from build123d import *

# Parameters (mm, degrees)
SKETCH1_R           = 5.2575
BOSS_EXTRUDE2_DEPTH = 18.3
SKETCH3_R           = 1.75
CUT_EXTRUDE2_DEPTH  = 19.8
SKETCH4_R           = 5.2575
SKETCH4_R_2         = 3.5
CUT_EXTRUDE3_DEPTH  = 16.5
FILLET1_R           = 0.5
FILLET2_R           = 0.25
FILLET3_R           = 0.5


with BuildPart() as part:
    # Sketch1 → Boss-Extrude2 (new body)
    with BuildSketch(Plane(origin=(0, 0, 0), x_dir=(1, 0, 0), z_dir=(0, 1, 0))):
        with Locations(Location((0, 0, 0), (0, 0, 270))):
            Circle(SKETCH1_R)
    extrude(amount=BOSS_EXTRUDE2_DEPTH)

    # Sketch3 → Cut-Extrude2 (cut)
    with BuildSketch(Plane(origin=(0, 0, 0), x_dir=(-1, 0, 0), z_dir=(0, -1, 0))):
        with Locations(Location((0, 0, 0), (0, 0, 90))):
            Circle(SKETCH3_R)
    extrude(amount=-CUT_EXTRUDE2_DEPTH, mode=Mode.SUBTRACT)

    # Sketch4 → Cut-Extrude3 (cut)
    with BuildSketch(Plane(origin=(0, 0, 0), x_dir=(-1, 0, 0), z_dir=(0, -1, 0))):
        with Locations(Location((0, 0, 0), (0, 0, 90))):
            Circle(SKETCH4_R)
        with Locations(Location((0, 0, 0), (0, 0, 90))):
            Circle(SKETCH4_R_2, mode=Mode.SUBTRACT)
    extrude(amount=-CUT_EXTRUDE3_DEPTH, mode=Mode.SUBTRACT)

    # Fillet1
    fillet1_edges = [part.edges().sort_by_distance(p)[0] for p in [
        (0, 18.3, -5.2575),
    ]]
    fillet(fillet1_edges, radius=FILLET1_R)

    # Fillet2
    fillet2_edges = [part.edges().sort_by_distance(p)[0] for p in [
        (0, 18.3, 1.75),
    ]]
    fillet(fillet2_edges, radius=FILLET2_R)

    # Fillet3
    fillet3_edges = [part.edges().sort_by_distance(p)[0] for p in [
        (0, 16.5, -5.2575),
    ]]
    fillet(fillet3_edges, radius=FILLET3_R)


solid = part.part
Geometry check sheet. Reference: the model listing, model coordinates, mm. Give positions to 0.01 mm unless a question says otherwise; leave off trailing zeros. Loops run counter-clockwise (first coordinate to the right, second up) from the corner with the lowest first, then second, coordinate; pieces in that order, holes last.
(1) Release check for a two-part mould opening along Z. For faces 1 (the cylindrical face through (-3.417, 8.134, 0.759)), 2 (the cylindrical face through (-1.71, 8.9, 0.38)), 3 (the flat face through (4, 16.5, 0)) record: released by +Z, released by -Z, zero draft, split by the parting line, or undercut.
From the geometry:
face 1: split by the parting line
face 2: undercut
face 3: zero draft
(2) Depth check by flat-ended pin: pin 1 Ø1 at (y, z) = (10, -2.5) entering from +X; pin 2 Ø3 at (x, z) = (0, 0) entering from +Y; pin 3 Ø1.5 at (y, z) = (14.5, 3.5) entering from -X; pin 4 Ø4 at (y, z) = (6.5, 2) entering from -X. Enter the tip coordinate at first touch or a pass-through.
From the geometry:
pin 1: stops at x = 2.87
pin 2: passes through
pin 3: stops at x = -2.17
pin 4: stops at x = -3.5
(3) Section check B-B on z = 0. Record the cut outline in (x, y), then the cut area to 3 significant figures.
From the geometry:
outline: (-5.26, 17) arc R0.5 ccw to (-4.76, 16.5) - (-3.5, 16.5) - (-3.5, 0) - (-1.75, 0) - (-1.75, 18.05) arc R0.25 ccw to (-2, 18.3) - (-4.76, 18.3) arc R0.5 ccw to (-5.26, 17.8) - close; (1.75, 0) - (3.5, 0) - (3.5, 16.5) - (4.76, 16.5) arc R0.5 ccw to (5.26, 17) - (5.26, 17.8) arc R0.5 ccw to (4.76, 18.3) - (2, 18.3) arc R0.25 ccw to (1.75, 18.05) - close
area: 70.1 mm2
(4) Section check C-C on y = 11. Record the cut outline in (x, z), then the cut area to 3 significant figures.
From the geometry:
outline: circle Ø7 at (0, 0); hole circle Ø3.5 at (0, 0)
area: 28.9 mm2
(5) Section check A-A on x = 0. Record the cut outline in (y, z).
From the geometry:
outline: (0, -3.5) - (16.5, -3.5) - (16.5, -4.76) arc R0.5 ccw to (17, -5.26) - (17.8, -5.26) arc R0.5 ccw to (18.3, -4.76) - (18.3, -2) arc R0.25 ccw to (18.05, -1.75) - (0, -1.75) - close; (0, 1.75) - (18.05, 1.75) arc R0.25 ccw to (18.3, 2) - (18.3, 4.76) arc R0.5 ccw to (17.8, 5.26) - (17, 5.26) arc R0.5 ccw to (16.5, 4.76) - (16.5, 3.5) - (0, 3.5) - close
(6) Thickness scan on L1, parallel to X at y = 4, z = 0; L2, parallel to Y at x = 0.75, z = 4.75; L3, parallel to X at y = 3.5, z = 1. Record the ranges inside material, lowest first.
From the geometry:
L1: x = -3.5 to -1.75, 1.75 to 3.5
L2: y = 16.5 to 18.3
L3: x = -3.35 to -1.44, 1.44 to 3.35
